Read the model definition and answer for the solid it produces. Units are mm, in the model's axes. A direction names the side the tool comes from. Coordinates: 2 decimals unless noted, no trailing zeros. Loops run counter-clockwise (first coordinate to the right, second up) from the corner with the lowest first, then second, coordinate; pieces in that order, holes last. Notation, with made-up numbers: (50.5, -20) -> (60.5, -20) arc R16 cw to (60.5, -7) -> close; hole circle Ø5 at (-35.75, 13). An arc over 180 degrees is marked (long way). Answer in a Markdown table with one row per item.
```python
from build123d import *

# Parameters (mm, degrees)
EXTRUDE_1_DEPTH      = 18.8
EXTRUDE_1_DEPTH_BACK = 1.2
SKETCH_1_R           = 6.6
CHAMFER_1_SIZE       = 0.5
SKETCH_2_R           = 2
CUT_EXTRUDE_1_DEPTH  = 13.4
SKETCH_3_R           = 1.5
CUT_EXTRUDE_2_DEPTH  = 13.4


with BuildPart() as part:
    # 草图1 → 凸台-拉伸1 (new, two sides: drawn at the far end of the back side and taken through both)
    with BuildSketch(Plane(origin=(0, 0, 0), x_dir=(1, 0, 0), z_dir=(0, 1, 0)).offset(-EXTRUDE_1_DEPTH_BACK)):
        with Locations(Location((0, 0, 0), (0, 0, 270))):
            Circle(SKETCH_1_R)
    extrude(amount=EXTRUDE_1_DEPTH + EXTRUDE_1_DEPTH_BACK)

    # 倒角1
    chamfer_1_edges = [part.edges().sort_by_distance(p)[0] for p in [
        (0, -1.2, -6.6),
        (0, 18.8, -6.6),
    ]]
    chamfer(chamfer_1_edges, length=CHAMFER_1_SIZE)

    # 草图2 → 切除-拉伸1 (cut)
    with BuildSketch(Plane(origin=(0, 18.8, 0), x_dir=(1, 0, 0), z_dir=(0, 1, 0))):
        with Locations(Location((0, 0, 0), (0, 0, 270))):
            Circle(SKETCH_2_R)
    extrude(amount=-CUT_EXTRUDE_1_DEPTH, mode=Mode.SUBTRACT)

    # 草图3 → 切除-拉伸2 (cut)
    with BuildSketch(Plane.XY):
        with Locations(Location((0, 15.8, 0), (0, 0, 90))):
            Circle(SKETCH_3_R)
    extrude(amount=CUT_EXTRUDE_2_DEPTH, mode=Mode.SUBTRACT)


solid = part.part
```
1. A cutting plane is placed at B-B on z = 0. Give the vertices of the cut face in (x, y).
A:
| item | result |
|---|---|
| outline | (-6.6, -0.7) -> (-6.1, -1.2) -> (6.1, -1.2) -> (6.6, -0.7) -> (6.6, 18.3) -> (6.1, 18.8) -> (2, 18.8) -> (2, 5.4) -> (-2, 5.4) -> (-2, 18.8) -> (-6.1, 18.8) -> (-6.6, 18.3) -> close |
2. A cutting plane is placed at C-C on y = 12.75. Give the vertices of the cut face in (x, z).
A:
| item | result |
|---|---|
| outline | circle Ø13.2 at (0, 0); hole circle Ø4 at (0, 0) |
3. A tool of negligible diameter and unlimited length cuts with its end or side. For faces 1 (the flat face through (0, 18.8, 3)), 2 (the flat face through (0, 5.4, 0)), 3 (the cylindrical face through (-0.45, 17.23, 3.92)), from which of +Z, -Z, +X, -X, +Y, -Y can it reach the whole face along a straight path? Write none if from no direction.
A:
| item | result |
|---|---|
| face 1 | +Z, -Z, +X, -X, +Y |
| face 2 | +Y |
| face 3 | +Z |
4. A cutting plane is placed at A-A on x = 0. Give the vertices of the cut face in (y, z).
A:
| item | result |
|---|---|
| outline | (-1.2, -6.1) -> (-0.7, -6.6) -> (18.3, -6.6) -> (18.8, -6.1) -> (18.8, -2) -> (5.4, -2) -> (5.4, 2) -> (14.3, 2) -> (14.3, 6.6) -> (-0.7, 6.6) -> (-1.2, 6.1) -> close; (17.3, 2) -> (18.8, 2) -> (18.8, 6.1) -> (18.3, 6.6) -> (17.3, 6.6) -> close |
5. Given pin 1 Ø1 at (x, y) = (2, 9) entering from +Z; pin 2 Ø1.8 at (x, y) = (0, 15.8) entering from +Z; pin 3 Ø4 at (y, z) = (10, -3) entering from -X, each flat-ended and moving along its own axis, determine where each tip first touches the part or whether it passes through.
A:
| item | result |
|---|---|
| pin 1 | stops at z = 6.43 |
| pin 2 | stops at z = -1.79 |
| pin 3 | stops at x = -6.52 |
6. Find the intervals of material crossed by probe 1 along Y at (x, z) = (0, 4.45); probe 2 along X at (y, z) = (13.75, 0); probe 3 along X at (y, z) = (15.8, 5), in increasing order.
A:
| item | result |
|---|---|
| probe 1 | y = -1.2 to 14.3, 17.3 to 18.8 |
| probe 2 | x = -6.6 to -2, 2 to 6.6 |
| probe 3 | x = -4.31 to -1.5, 1.5 to 4.31 |
7. A cutting plane is placed at D-D on y = 15.8. Give the vertices of the cut face in (x, z), and give its area (3 significant figures).
A:
| item | result |
|---|---|
| outline | (-1.5, 1.32) -> (-1.5, 6.43) arc R6.6 ccw (long way) to (1.5, 6.43) -> (1.5, 1.32) arc R2 cw (long way) to start |
| area | 110 mm2 |
8. The mould has two halves that part along X. Classify faces 4 (the flat face through (0, -1.2, 0)), 5 (the cylindrical face through (-4.016, 8.667, -5.238)), 6 (the cylindrical face through (0, 12, -2)): pulls with the +X half, pulls with the -X half, needs draft (parallel to the pull), parting line crosses it, or undercut.
A:
| item | result |
|---|---|
| face 4 | needs draft |
| face 5 | parting line crosses it |
| face 6 | undercut |
